Check sheet for the modelled part. Datum: model origin and axes. Units: mm. Give positions to 0.01 mm unless a question says otherwise; leave off trailing zeros. Write each loop counter-clockwise with the first axis right and the second up, starting at its lowest first coordinate (ties: lowest second). Pieces come first, ordered by that corner, then holes. Notation, with made-up numbers: (0.25, 17.5) -> (43.25, 17.5) arc R16 ccw to (43.25, 44.5) -> close; hole circle Ø6 at (-26.75, 49). An arc over 180 degrees is marked (long way). Answer as a JSON object with one key per item and string values.
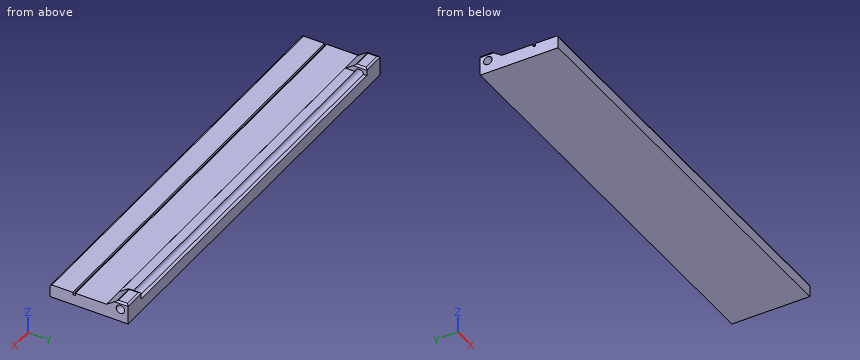
from build123d import *

# Parameters (mm, degrees)
SKETCH_R     = 2.5
PAD_DEPTH    = 248
SKETCH001_W  = 4.639466
SKETCH001_H  = 222.6
POCKET_DEPTH = 25.4
FILLET_R     = 1
FILLET001_R  = 1
FILLET002_R  = 1


with BuildPart() as part:
    # Sketch → Pad (new body)
    with BuildSketch(Plane.YZ):
        Polygon((0, 0), (45.8, 0), (45.8, 7.62), (45.8, 11.938), (39.266743, 11.938), (33.1, 7.62), (14.8, 7.62), (14.8, 6.12), (13.3, 6.12), (13.3, 7.62), (0, 7.62), align=None)
        with Locations((41.3, 7.438)):
            Circle(SKETCH_R, mode=Mode.SUBTRACT)
    extrude(amount=PAD_DEPTH)

    # Sketch001 (on Face3 of Pad) → Pocket (cut)
    with BuildSketch(Plane.ZX.offset(45.8)):
        with Locations((9.990006, 124)):
            Rectangle(SKETCH001_W, SKETCH001_H)
    extrude(amount=-POCKET_DEPTH, mode=Mode.SUBTRACT)

    # Fillet
    fillet_edges = [part.edges().sort_by_distance(p)[0] for p in [
        (124, 0, 7.62),
    ]]
    fillet(fillet_edges, radius=FILLET_R)

    # Fillet001
    fillet001_edges = [part.edges().sort_by_distance(p)[0] for p in [
        (235.3, 42.533372, 11.938),
        (241.65, 39.266743, 11.938),
        (248, 42.533372, 11.938),
        (241.65, 45.8, 11.938),
    ]]
    fillet(fillet001_edges, radius=FILLET001_R)

    # Fillet002
    fillet002_edges = [part.edges().sort_by_distance(p)[0] for p in [
        (0, 42.533372, 11.938),
        (6.35, 39.266743, 11.938),
        (12.7, 42.533372, 11.938),
        (6.35, 45.8, 11.938),
    ]]
    fillet(fillet002_edges, radius=FILLET002_R)


solid = part.part
1. Scan lines: L1, parallel to Y at x = 187, z = 7.5; L2, parallel to Z at x = 81.5, y = 34.5; L3, parallel to Z at x = 62.5, y = 41.3. Record each from-to range of solid material in increasing order. Write a range as [from, to].
Determined:
{"L1": "[0.53, 13.3], [14.8, 38.8], [43.8, 45.8]", "L2": "[0, 7.67]", "L3": "[0, 4.94]"}
2. Sectioned sample at A-A, the plane x = 33.5. Enter the section's corners in (y, z), plus the area to 3 significant figures.
Determined:
{"outline": "(0, 0) -> (45.8, 0) -> (45.8, 7.67) -> (43.79, 7.67) arc R2.5 cw (long way) to (38.81, 7.67) -> (33.17, 7.67) -> (33.1, 7.62) -> (14.8, 7.62) -> (14.8, 6.12) -> (13.3, 6.12) -> (13.3, 7.62) -> (1, 7.62) arc R1 ccw to (0, 6.62) -> close", "area": "336 mm^2"}
3. Go/stop test with flat-tipped pins: P1, Ø10, axis at x = 149.5, y = 17, coming from the +Z side; P2, Ø6, axis at x = 99, y = 35.5, coming from the +Z side; P3, Ø0.8, axis at x = 97, y = 14, coming from the +Z side. Record where each tip stops, or that it passes through.
Determined:
{"P1": "z = 7.62", "P2": "z = 7.67", "P3": "z = 6.12"}
